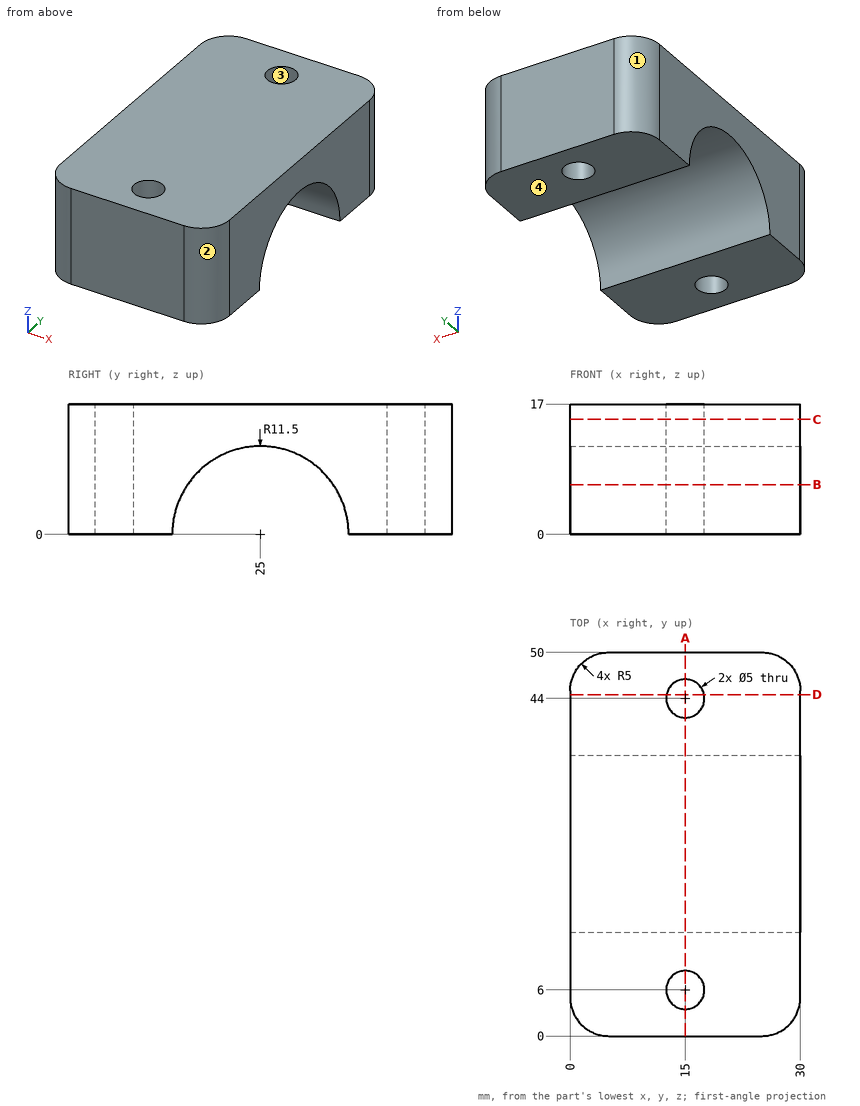
Study the drawing (mm; zero at the part's minimum x, y, z) and answer. Give positions to 0.01 mm unless a question says otherwise; leave off trailing zeros. Order: outer loops, then holes, each group sorted by start corner. A loop starts at its lowest first (then second) coordinate and runs counter-clockwise, first axis right, second up. Notation, with made-up numbers: M -2,73 L 45,73 A18 cw 45,79 Z; hole C 76,-7.5 d9. An arc over 180 degrees is marked long. Put each result on its own line as item: value. Start each with the question number.
Item 1: For a pull along X with two mould halves and no side action, classify the marked faces 1, 2, 3 and 4 as +X half, -X half, draft (parallel to the pull), parting line (faces both ways), or undercut.
Item 2: The part is cut by section A-A, the plane x = 15. Determine the outline of the cut face in (y, z).
Item 3: The part is cut by section C-C, the plane z = 15. Determine the outline of the cut face in (x, y).
Item 4: The part is cut by section B-B, the plane z = 6.5. Determine the outline of the cut face in (x, y).
Item 5: The part is cut by section D-D, the plane y = 44.5. Determine the outline of the cut face in (x, z), and give its area (3 significant figures).
Item 6: Flat-ended cylindrical pins translate along their axes: P1, Ø6, axis at y = 25.5, z = 10.5, coming from the +X side; P2, Ø3, axis at x = 25, y = 26.5, coming from the -Z side; P3, Ø1.5, axis at x = 3, z = 10, coming from the -Y side. Find the tip coordinate at first contact, or state that the pin passes through.
Item 7: Find the intervals of material crossed by line 1 along X through (y, z) = (44, 6); line 2 along Y through (x, z) = (15, 4); line 3 along Y through (x, z) = (15, 5.5), in increasing order.
Answer key:
1. face 1: -X half
1. face 2: +X half
1. face 3: undercut
1. face 4: draft
2. outline: M 0,0 L 3.5,0 L 3.5,17 L 0,17 Z; M 8.5,0 L 13.5,0 A11.5 cw 36.5,0 L 41.5,0 L 41.5,17 L 8.5,17 Z; M 46.5,0 L 50,0 L 50,17 L 46.5,17 Z
3. outline: M 0,5 A5 ccw 5,0 L 25,0 A5 ccw 30,5 L 30,45 A5 ccw 25,50 L 5,50 A5 ccw 0,45 Z; hole C 15,6 d5; hole C 15,44 d5
4. outline: M 0,5 A5 ccw 5,0 L 25,0 A5 ccw 30,5 L 30,15.51 L 0,15.51 Z; M 0,34.49 L 30,34.49 L 30,45 A5 ccw 25,50 L 5,50 A5 ccw 0,45 Z; hole C 15,6 d5; hole C 15,44 d5
5. outline: M 0,0 L 12.55,0 L 12.55,17 L 0,17 Z; M 17.45,0 L 30,0 L 30,17 L 17.45,17 Z
5. area: 427 mm²
6. P1: stops at x = 30
6. P2: stops at z = 11.1
6. P3: stops at y = 0.16
7. line 1: x = 0 to 12.5, 17.5 to 30
7. line 2: y = 0 to 3.5, 8.5 to 14.22, 35.78 to 41.5, 46.5 to 50
7. line 3: y = 0 to 3.5, 8.5 to 14.9, 35.1 to 41.5, 46.5 to 50
